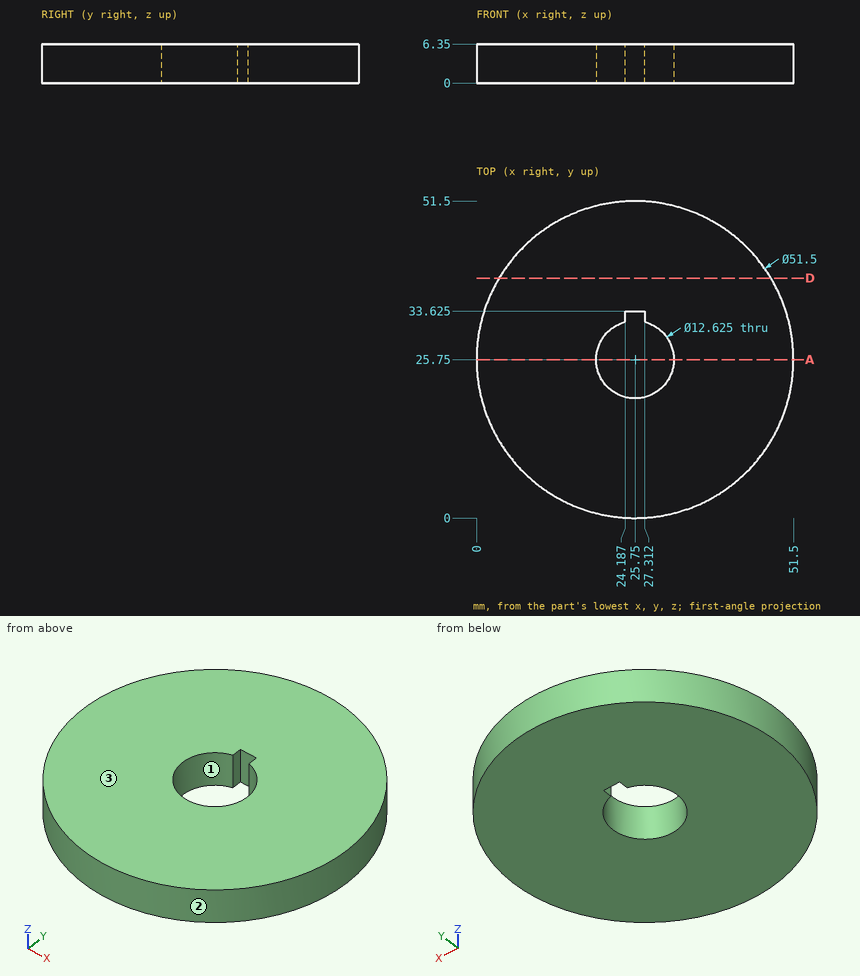
Part print with two shaded views. Sizes in mm from the minimum x, y, z corner. Round coordinates to 2 decimals unless told otherwise and drop trailing zeros. Loops run counter-clockwise (first coordinate to the right, second up) from the corner with the lowest first, then second, coordinate; pieces in that order, holes last. Notation, with made-up numbers: (63, 69.5) - (116, 69.5) arc R23 cw to (116, 85.5) - close; hole circle Ø4 at (57.5, 20.5). An arc over 180 degrees is marked (long way). Put each result on its own line as item: value.
1. Slice it at D-D on y = 39. List the corners of the cut face in (x, z).
Geometry check:
outline: (3.67, 0) - (47.83, 0) - (47.83, 6.35) - (3.67, 6.35) - close
2. Slice it at A-A on y = 25.75. List the corners of the cut face in (x, z).
Geometry check:
outline: (0, 0) - (19.44, 0) - (19.44, 6.35) - (0, 6.35) - close; (32.06, 0) - (51.5, 0) - (51.5, 6.35) - (32.06, 6.35) - close
3. Two-plate mould, pull along X, no slides. Class the marked faces 1, 2 and 3: released by +X, released by -X, zero draft, split by the parting line, or undercut.
Geometry check:
face 1: undercut
face 2: split by the parting line
face 3: zero draft
4. Pin check, flat tips, straight feed: P1, Ø2.5, axis at x = 26.5, z = 2.5, coming from the -Y side; P2, Ø0.9, axis at y = 33, z = 3, coming from the +X side (1 decimal); P3, Ø1.4, axis at y = 33, z = 3.5, coming from the -X side. Stop position of each tip, or through.
Geometry check:
P1: y = 0
P2: x = 50.6
P3: x = 0.85
5. Wall check: line 1 (Y direction, x = 25.75, z = 4.75) (1 decimal); line 2 (Y direction, x = 31, z = 5.75) (1 decimal); line 3 (X direction, y = 9.5, z = 3) (1 decimal). Give the ranges that are in metal, low to high.
Geometry check:
line 1: 0 to 19.4, 33.6 to 51.5
line 2: 0.5 to 22.2, 29.3 to 51
line 3: 5.8 to 45.7
